from build123d import *

# Parameters (mm, degrees)
F0_R     = 35
F0_R_2   = 1.5
F0_W     = 19.983293198
F0_H     = 32
F1_DEPTH = 2


# Not quite as in the source:
# - a feature names something its author has since deleted; it is built from what else it names


with BuildPart() as f1:
    # F0 (on Top) → F1 (new body)
    with BuildSketch(Plane.XY):
        Circle(F0_R)
        with Locations((0, -32.5)):
            Circle(F0_R_2, mode=Mode.SUBTRACT)
        with Locations((-32.5, 0)):
            Circle(F0_R_2, mode=Mode.SUBTRACT)
        with BuildLine():
            ThreePointArc((29.7321374946, 4), (29.9329594664, 2.0044793789), (30, 0))
            ThreePointArc((30, 0), (29.9329594664, -2.0044793789), (29.7321374946, -4))
            ThreePointArc((29.7321374946, -4), (21.2132034356, -21.2132034356), (4, -29.7321374946))
            ThreePointArc((4, -29.7321374946), (0, -30), (-4, -29.7321374946))
            ThreePointArc((-4, -29.7321374946), (-21.2132034356, -21.2132034356), (-29.7321374946, -4))
            ThreePointArc((-29.7321374946, -4), (-30, 0), (-29.7321374946, 4))
            ThreePointArc((-29.7321374946, 4), (-21.2132034356, 21.2132034356), (-4, 29.7321374946))
            ThreePointArc((-4, 29.7321374946), (0, 30), (4, 29.7321374946))
            ThreePointArc((4, 29.7321374946), (21.2132034356, 21.2132034356), (29.7321374946, 4))
        make_face(mode=Mode.SUBTRACT)
        with Locations((32.5, 0)):
            Circle(F0_R_2, mode=Mode.SUBTRACT)
        with Locations((0, 32.5)):
            Circle(F0_R_2, mode=Mode.SUBTRACT)
        with BuildLine():
            Line((4, 18), (4, 29.7321374946))
            ThreePointArc((4, 29.7321374946), (0, 30), (-4, 29.7321374946))
            Line((-4, 29.7321374946), (-4, 18))
            Line((-4, 18), (4, 18))
        make_face()
        with BuildLine():
            Line((-12, 4), (-29.7321374946, 4))
            ThreePointArc((-29.7321374946, 4), (-30, 0), (-29.7321374946, -4))
            Line((-29.7321374946, -4), (-12, -4))
            Line((-12, -4), (-12, 4))
        make_face()
        with BuildLine():
            ThreePointArc((-4, -29.7321374946), (0, -30), (4, -29.7321374946))
            Line((4, -29.7321374946), (4, -18))
            Line((4, -18), (-4, -18))
            Line((-4, -18), (-4, -29.7321374946))
        make_face()
        Polygon((12, -4), (12, 4), (12, 12.1005004627), (12, 18), (4, 18), (-4, 18), (-12, 18), (-12, 4), (-12, -4), (-12, -18), (-4, -18), (4, -18), (12, -18), (12, -5.151443038), align=None)
        with Locations((0.1530251862, 0.242334145)):
            Rectangle(F0_W, F0_H, mode=Mode.SUBTRACT)
        with Locations((0.1530251862, 0.242334145)):
            Rectangle(F0_W, F0_H)
        with BuildLine():
            ThreePointArc((29.7321374946, -4), (29.9329594664, -2.0044793789), (30, 0))
            ThreePointArc((30, 0), (29.9329594664, 2.0044793789), (29.7321374946, 4))
            Line((29.7321374946, 4), (12, 4))
            Line((12, 4), (12, -4))
            Line((12, -4), (29.7321374946, -4))
        make_face()
    extrude(amount=F1_DEPTH)


solid = f1.part
Input: part model. Units: mm. Frame: model coordinates. Give positions to 0.01 mm unless a question says otherwise; leave off trailing zeros. Order: outer loops, then holes, each group sorted by start corner. A loop starts at its lowest first (then second) coordinate and runs counter-clockwise, first axis right, second up. Notation, with made-up numbers: (11.25, 50.25) -> (35.25, 50.25) arc R18 cw to (35.25, 64.25) -> close; hole circle Ø7 at (1, 36.25). An arc over 180 degrees is marked (long way). Use one line per item in the form item = value.
1) Section B-B, the plane y = -8. Return loops of the section in (x, z).
Response values:
outline = (-34.07, 0) -> (-28.91, 0) -> (-28.91, 2) -> (-34.07, 2) -> close; (-12, 0) -> (12, 0) -> (12, 2) -> (-12, 2) -> close; (28.91, 0) -> (34.07, 0) -> (34.07, 2) -> (28.91, 2) -> close
2) Section A-A, the plane x = 0. Return loops of the section in (y, z).
Response values:
outline = (-35, 0) -> (-34, 0) -> (-34, 2) -> (-35, 2) -> close; (-31, 0) -> (31, 0) -> (31, 2) -> (-31, 2) -> close; (34, 0) -> (35, 0) -> (35, 2) -> (34, 2) -> close
3) Mould query, pull axis Y, two halves, no side actions, for faces 1 (the flat face through (0, 0, 2)), 2 (the flat face through (12, 11, 1)). Classes: pulls with the +Y half, pulls with the -Y half, needs draft (parallel to the pull), parting line crosses it, or undercut.
Response values:
face_1 = needs draft
face_2 = undercut
4) Section C-C, the plane z = 1.15. Count the separate pieces of the cut face and the enclosed holes in it, and give its area (3 significant figures).
Response values:
separate_pieces = 1
enclosed_holes = 8
area = 2,330 mm^2
5) First-contact query: pin 1 Ø1.8 at (x, y) = (0, -32.5) entering from -Z (1 decimal); pin 2 Ø0.6 at (x, z) = (-24.5, 1) entering from +Y; pin 3 Ø0.6 at (y, z) = (25.5, 1) entering from +X; pin 4 Ø0.6 at (y, z) = (-11.5, 1.5) entering from +X. Flat tips, straight axial feed; report the tip coordinate or a pass-through.
Response values:
pin_1 = through
pin_2 = 25.29
pin_3 = 24.29
pin_4 = 33.16
6) Section D-D, the plane x = -32.5. Return loops of the section in (y, z), and give its area (3 significant figures).
Response values:
outline = (-12.99, 0) -> (-1.5, 0) -> (-1.5, 2) -> (-12.99, 2) -> close; (1.5, 0) -> (12.99, 0) -> (12.99, 2) -> (1.5, 2) -> close
area = 46.0 mm^2
7) Line query: probe 1 along Y at (x, z) = (0, 0.85); probe 2 along X at (y, z) = (-27, 0.95); probe 3 along Y at (x, z) = (9, 0.55). Output: solid intervals per line, ascending.
Response values:
probe_1 = -35 to -34, -31 to 31, 34 to 35
probe_2 = -22.27 to -13.08, -4 to 4, 13.08 to 22.27
probe_3 = -33.82 to -28.62, -18 to 18, 28.62 to 33.82
